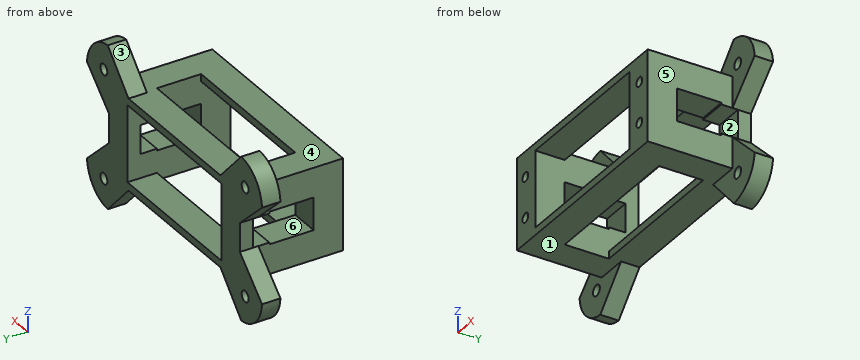
from build123d import *

# Parameters (mm, degrees)
SKETCH2_W               = 57.2
SKETCH2_H               = 24.8
SKETCH2_W_2             = 41.2
SKETCH2_H_2             = 20.8
BOSS_EXTRUDE2_DEPTH     = 28
SKETCH4_W               = 8.8
SKETCH4_H               = 12
CUT_EXTRUDE1_DEPTH      = 73
SKETCH5_W               = 41.2
SKETCH5_H               = 12
CUT_EXTRUDE2_DEPTH      = 28
SKETCH6_R               = 1.25
CUT_EXTRUDE3_DEPTH      = 7
SKETCH7_R               = 1.5
BOSS_EXTRUDE3_DEPTH     = 5
MIRROR2_COPY_1_SKETCH_R = 1.5
MIRROR2_COPY_1_DEPTH    = 5
BOSS_EXTRUDE4_START     = -5
BOSS_EXTRUDE4_DEPTH     = 5
MIRROR4_START           = -5
MIRROR4_COPY_1_DEPTH    = 5
CUT_EXTRUDE4_DEPTH      = 80.302431776


with BuildPart() as part:
    # Sketch2 → Boss-Extrude2 (new body)
    with BuildSketch(Plane.XZ):
        with Locations((0, -10)):
            Rectangle(SKETCH2_W, SKETCH2_H)
        with Locations((0, -10)):
            Rectangle(SKETCH2_W_2, SKETCH2_H_2, mode=Mode.SUBTRACT)
    extrude(amount=BOSS_EXTRUDE2_DEPTH)

    # Sketch4 → Cut-Extrude1 (cut)
    with BuildSketch(Plane.ZY.offset(28.6)):
        with Locations((-10, -14)):
            Rectangle(SKETCH4_W, SKETCH4_H)
    extrude(amount=-CUT_EXTRUDE1_DEPTH, mode=Mode.SUBTRACT)

    # Sketch5 → Cut-Extrude2 (cut)
    with BuildSketch(Plane.XY.offset(2.4)):
        with Locations((0, -14)):
            Rectangle(SKETCH5_W, SKETCH5_H)
    extrude(amount=-CUT_EXTRUDE2_DEPTH, mode=Mode.SUBTRACT)

    # Sketch6 → Cut-Extrude3 (cut)
    with BuildSketch(Plane.XZ.offset(28)):
        with Locations((-24.929249083, -15.5)):
            Circle(SKETCH6_R)
        with Locations((-24.929249083, -4.5)):
            Circle(SKETCH6_R)
        with Locations((24.929249083, -15.5)):
            Circle(SKETCH6_R)
        with Locations((24.929249083, -4.5)):
            Circle(SKETCH6_R)
    extrude(amount=-CUT_EXTRUDE3_DEPTH, mode=Mode.SUBTRACT)

    # Sketch7 → Boss-Extrude3 (add)
    with BuildSketch(Plane(origin=(0, 0, 0), x_dir=(1, 0, 0), z_dir=(0, 1, 0))):
        with BuildLine():
            Line((-28.6, -2.4), (-28.6, 0.6))
            Line((-28.6, 0.6), (-33.943490451, -4.423862881))
            ThreePointArc((-33.943490451, -4.423862881), (-32.636549964, -6.444153255), (-30.613803719, -7.74728957))
            Line((-30.613803719, -7.74728957), (-25.6, -2.4))
            Line((-25.6, -2.4), (-28.6, -2.4))
        make_face()
        with Locations(Location((-30.9, -4.7, 0), (0, 0, 180))):
            Circle(SKETCH7_R, mode=Mode.SUBTRACT)
    boss_extrude3 = extrude(amount=-BOSS_EXTRUDE3_DEPTH)

    # Mirror1: Boss-Extrude3 across plane
    add(boss_extrude3.mirror(Plane.ZY))

    # Mirror2: Boss-Extrude3 across plane
    add(boss_extrude3.mirror(Plane.XY.offset(-10)))

    # Mirror2 copy 1 sketch → Mirror2 copy 1 (add)
    with BuildSketch(Plane(origin=(0, 0, -20), x_dir=(-1, 0, 0), z_dir=(0, 1, 0))):
        with BuildLine():
            Line((-28.6, -2.4), (-28.6, 0.6))
            Line((-28.6, 0.6), (-33.943490451, -4.423862881))
            ThreePointArc((-33.943490451, -4.423862881), (-32.636549964, -6.444153255), (-30.613803719, -7.74728957))
            Line((-30.613803719, -7.74728957), (-25.6, -2.4))
            Line((-25.6, -2.4), (-28.6, -2.4))
        make_face()
        with Locations(Location((-30.9, -4.7, 0), (0, 0, 180))):
            Circle(MIRROR2_COPY_1_SKETCH_R, mode=Mode.SUBTRACT)
    extrude(amount=-MIRROR2_COPY_1_DEPTH)

    # Sketch8 → Boss-Extrude4 (add)
    with BuildSketch(Plane.XZ.offset(5).offset(BOSS_EXTRUDE4_START)):
        with BuildLine():
            Line((28.6, -0.6), (28.6, -6.090275739))
            Line((28.6, -6.090275739), (38.293875859, 3.023748801))
            ThreePointArc((38.293875859, 3.023748801), (35.462849129, 9.2747068), (29.207013206, 12.0949382))
            Line((29.207013206, 12.0949382), (20.116703701, 2.4))
            Line((20.116703701, 2.4), (25.6, 2.4))
            Line((25.6, 2.4), (30.613803719, 7.74728957))
            ThreePointArc((30.613803719, 7.74728957), (32.636549964, 6.444153255), (33.943490451, 4.423862881))
            Line((33.943490451, 4.423862881), (28.6, -0.6))
        make_face()
    boss_extrude4 = extrude(amount=BOSS_EXTRUDE4_DEPTH)

    # Mirror3: Boss-Extrude4 across plane
    add(boss_extrude4.mirror(Plane(origin=(0, 0, -10), x_dir=(1, 0, 0), z_dir=(0, 0, -1))))

    # Mirror4: Boss-Extrude4 across plane
    add(boss_extrude4.mirror(Plane.ZY))

    # Mirror4 copy 1 sketch → Mirror4 copy 1 (add)
    with BuildSketch(Plane(origin=(0, -5, -20), x_dir=(-1, 0, 0), z_dir=(0, -1, 0)).offset(MIRROR4_START)):
        with BuildLine():
            Line((28.6, -0.6), (28.6, -6.090275739))
            Line((28.6, -6.090275739), (38.293875859, 3.023748801))
            ThreePointArc((38.293875859, 3.023748801), (35.462849129, 9.2747068), (29.207013206, 12.0949382))
            Line((29.207013206, 12.0949382), (20.116703701, 2.4))
            Line((20.116703701, 2.4), (25.6, 2.4))
            Line((25.6, 2.4), (30.613803719, 7.74728957))
            ThreePointArc((30.613803719, 7.74728957), (32.636549964, 6.444153255), (33.943490451, 4.423862881))
            Line((33.943490451, 4.423862881), (28.6, -0.6))
        make_face()
    extrude(amount=MIRROR4_COPY_1_DEPTH)

    # Sketch10 → Cut-Extrude4 (cut, through all)
    with BuildSketch(Plane(origin=(28.6, 0, 0), x_dir=(0, 0, -1), z_dir=(1, 0, 0))):
        Polygon((13.909724261, -5), (13.909724261, -3.5), (10, -3.5), (6.090275739, -3.5), (6.090275739, -5), (6.090275739, -8), (13.909724261, -8), align=None)
    extrude(amount=-CUT_EXTRUDE4_DEPTH, mode=Mode.SUBTRACT)


solid = part.part
Geometry check sheet. Reference: the model listing, model coordinates, mm. Face numbers are marked on the shaded views. A direction names the side the tool comes from. Give positions to 0.01 mm unless a question says otherwise; leave off trailing zeros. Write each loop counter-clockwise with the first axis right and the second up, starting at its lowest first coordinate (ties: lowest second). Pieces come first, ordered by that corner, then holes. Notation, with made-up numbers: (47, -18) - (70, -18) arc R34 cw to (70, 15) - close; hole circle Ø5 at (-27.75, 76). An arc over 180 degrees is marked (long way). Put each result on its own line as item: value.
1. Go/stop test with flat-tipped pins: pin 1 (12 mm diameter, centred on x = -18.5, y = -7.5, fed in from -Z); pin 2 (1.2 mm diameter, centred on x = 25, z = -16, fed in from -Y); pin 3 (12 mm diameter, centred on y = -4, z = -16.5, fed in from +X). Record where each tip stops, or that it passes through.
Ans:
pin 1: stops at z = -26.49
pin 2: stops at y = -21
pin 3: stops at x = 37.74
2. Thickness scan on line 1 (Z direction, x = -19, y = -1.75); line 2 (Z direction, x = 31.5, y = -4.5); line 3 (X direction, y = -16, z = -17). Record the ranges inside material, lowest first.
Ans:
line 1: z = -22.4 to -20.4, 0.4 to 2.4
line 2: z = -31.67 to -26.07, -23.33 to -16.64, -3.36 to 3.33, 6.07 to 11.67
line 3: x = -28.6 to -20.6, 20.6 to 28.6
3. Sectioned sample at B-B, the plane x = -19. Enter the section's corners in (y, z).
Ans:
outline: (-28, -22.4) - (-20, -22.4) - (-20, -20.4) - (-28, -20.4) - close; (-28, 0.4) - (-20, 0.4) - (-20, 2.4) - (-28, 2.4) - close; (-8, -22.4) - (0, -22.4) - (0, -20.4) - (-8, -20.4) - close; (-8, 0.4) - (0, 0.4) - (0, 2.4) - (-8, 2.4) - close
4. Sectioned sample at A-A, the plane y = -15.5. Enter the section's corners in (x, z), plus the area to 3 significant figures.
Ans:
outline: (-28.6, -22.4) - (-20.6, -22.4) - (-20.6, -14.4) - (-28.6, -14.4) - close; (-28.6, -5.6) - (-20.6, -5.6) - (-20.6, 2.4) - (-28.6, 2.4) - close; (20.6, -22.4) - (28.6, -22.4) - (28.6, -14.4) - (20.6, -14.4) - close; (20.6, -5.6) - (28.6, -5.6) - (28.6, 2.4) - (20.6, 2.4) - close
area: 256 mm²
5. Sectioned sample at D-D, the plane z = -4.5. Enter the section's corners in (x, y).
Ans:
outline: (-30.29, -5) - (-28.6, -5) - (-28.6, -28) - (-26.18, -28) - (-26.18, -21) - (-23.68, -21) - (-23.68, -28) - (-20.6, -28) - (-20.6, 0) - (-30.29, 0) - close; (20.6, -28) - (23.68, -28) - (23.68, -21) - (26.18, -21) - (26.18, -28) - (28.6, -28) - (28.6, -5) - (30.29, -5) - (30.29, 0) - (20.6, 0) - close
6. Set-up check for the marked faces 1, 2, 3 and 4: record each of +Z, -Z, +X, -X, +Y, -Y from which the full face is reachable in a straight line by a thin tool's end or side.
Ans:
face 1: -Z, -Y
face 2: +X, -X
face 3: +Z, +Y, -Y
face 4: +Z, -Y
7. Draft check along Y on the marked faces 5 and 6. Enter one of: +Y half, -Y half, draft (parallel to the pull), parting line (faces both ways), or undercut.
Ans:
face 5: draft
face 6: undercut
8. Sectioned sample at C-C, the plane y = -6.25. Enter the section's corners in (x, z), plus the area to 3 significant figures.
Ans:
outline: (-28.6, -22.4) - (28.6, -22.4) - (28.6, -13.91) - (20.6, -13.91) - (20.6, -20.4) - (-20.6, -20.4) - (-20.6, -13.91) - (-28.6, -13.91) - close; (-28.6, -6.09) - (-20.6, -6.09) - (-20.6, 0.4) - (20.6, 0.4) - (20.6, -6.09) - (28.6, -6.09) - (28.6, 2.4) - (-28.6, 2.4) - close
area: 436 mm²
